Could you check a few things on this model? Use its own coordinates, in mm. Give positions to 0.01 mm unless a question says otherwise; leave off trailing zeros. Order: outer loops, then holes, each group sorted by start corner. A loop starts at its lowest first (then second) coordinate and runs counter-clockwise, first axis right, second up. Notation, with made-up numbers: (31, 70.25) - (75, 70.25) arc R17 ccw to (75, 88.25) - close; hole circle Ø4 at (83, 49). An arc over 180 degrees is marked (long way). One line per question, with ' | ' between items. Start each with the question number.
1. I need wall thicknesses on probe 1 along X at (y, z) = (-84.5, 14.25); probe 2 along Z at (x, y) = (-1.5, -66.5); probe 3 along Y at (x, z) = (4, 10.25). Which ranges of each line are inside material? Lowest first, please. Write a range as from..to.
2. Imagine slicing it at D-D (y = -68). Please give me the cut outline in (x, z).
3. Imagine slicing it at C-C (z = 10). Give the number of separate pieces and of enclosed holes in the cut face, and give its area (3 significant figures).
4. Imagine slicing it at B-B (y = 90). Please give me the cut outline in (x, z), and give its area (3 significant figures).
5. Imagine slicing it at A-A (x = 1.25). Please give me the cut outline in (y, z).
```python
from build123d import *

# Parameters (mm, degrees)
SKETCH1_W           = 10
SKETCH1_H           = 200
BOSS_EXTRUDE1_DEPTH = 20
SHELL1_T            = -2
CUT_EXTRUDE1_DEPTH  = 10
SKETCH4_R           = 4
CUT_EXTRUDE3_DEPTH  = 10
SKETCH5_R           = 4
SKETCH5_R_2         = 3.5
CUT_EXTRUDE4_DEPTH  = 10


with BuildPart() as part:
    # Sketch1 → Boss-Extrude1 (new body)
    with BuildSketch(Plane.XY):
        Rectangle(SKETCH1_W, SKETCH1_H)
    extrude(amount=BOSS_EXTRUDE1_DEPTH)

    # Shell1
    shell1_openings = [part.faces().sort_by_distance(p)[0] for p in [
        (0, 100, 10),
        (0, -100, 10),
    ]]
    offset(amount=SHELL1_T, openings=shell1_openings, kind=Kind.INTERSECTION)

    # Sketch2 → Cut-Extrude1 (cut)
    with BuildSketch(Plane.ZY.offset(5)):
        Polygon((0, -100), (20, -80), (20, -100), align=None)
    extrude(amount=-CUT_EXTRUDE1_DEPTH, mode=Mode.SUBTRACT)

    # Sketch4 → Cut-Extrude3 (cut)
    with BuildSketch(Plane(origin=(5, 0, 0), x_dir=(0, 0, -1), z_dir=(1, 0, 0))):
        with Locations((-10, 90)):
            Circle(SKETCH4_R)
    extrude(amount=-CUT_EXTRUDE3_DEPTH, mode=Mode.SUBTRACT)

    # Sketch5 → Cut-Extrude4 (cut)
    with BuildSketch(Plane(origin=(5, 0, 0), x_dir=(0, 0, -1), z_dir=(1, 0, 0))):
        with Locations((-9.453331646, -76.40453273)):
            Circle(SKETCH5_R)
        with Locations((-10.347176909, -49.772000632)):
            Circle(SKETCH5_R_2)
    extrude(amount=-CUT_EXTRUDE4_DEPTH, mode=Mode.SUBTRACT)


solid = part.part
```
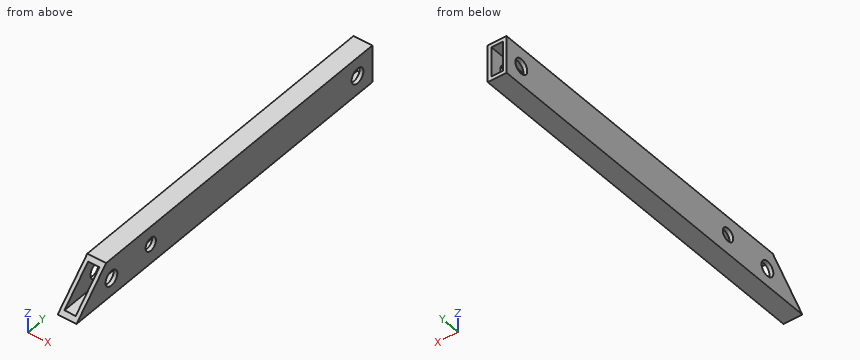
Results found:
1) probe 1: x = -5..-3, 3..5 | probe 2: z = 0..2, 18..20 | probe 3: y = -89.75..-80.32, -72.48..-53.27, -46.27..86.01, 93.99..100
2) outline: (-5, 0) - (5, 0) - (5, 20) - (-5, 20) - close; hole (-3, 2) - (3, 2) - (3, 18) - (-3, 18) - close
3) separate pieces: 8 | enclosed holes: 0 | area: 668 mm2
4) outline: (-5, 0) - (5, 0) - (5, 6) - (3, 6) - (3, 2) - (-3, 2) - (-3, 6) - (-5, 6) - close; (-5, 14) - (-3, 14) - (-3, 18) - (3, 18) - (3, 14) - (5, 14) - (5, 20) - (-5, 20) - close | area: 72.0 mm2
5) outline: (-100, 0) - (100, 0) - (100, 2) - (-98, 2) - close; (-82, 18) - (100, 18) - (100, 20) - (-80, 20) - close
